Input: part model. Units: mm. Frame: model coordinates. Give positions to 0.01 mm unless a question says otherwise; leave off trailing zeros. Loops run counter-clockwise (first coordinate to the right, second up) from the corner with the lowest first, then second, coordinate; pieces in that order, holes last. Notation, with made-up numbers: (-28.5, 47.5) -> (-15.5, 47.5) arc R16 cw to (-15.5, 58.5) -> close; hole circle Ø10 at (59.5, -34.5). An arc over 180 degrees is marked (long way). Use CSV: the item, a comma, the result in double quotes.
```python
from build123d import *

# Parameters (mm, degrees)
F1_DEPTH = 18
F2_W     = 640.407225
F2_H     = 6
F3_DEPTH = 6


with BuildPart() as f1:
    # F0 (on Top) → F1 (new body)
    with BuildSketch(Plane.XY):
        Polygon((322.5, -311), (322.5, 311), (-322.5, 311), (-84.441184, -311), align=None)
    extrude(amount=F1_DEPTH)

    # F2 (on face) → F3 (cut)
    with BuildSketch(Plane.XY.offset(18)):
        with Locations((2.296388, 296)):
            Rectangle(F2_W, F2_H)
    extrude(amount=-F3_DEPTH, mode=Mode.SUBTRACT)


solid = f1.part
```
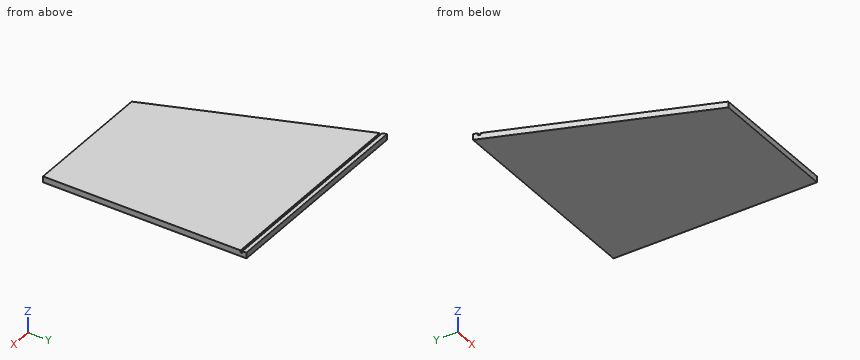
1) Section query A-A (x = -242). Return loops of the section in (y, z).
From the geometry:
outline,"(100.67, 0) -> (311, 0) -> (311, 18) -> (299, 18) -> (299, 12) -> (293, 12) -> (293, 18) -> (100.67, 18) -> close"
2) Section query C-C (y = -79). Return loops of the section in (x, z).
From the geometry:
outline,"(-173.23, 0) -> (322.5, 0) -> (322.5, 18) -> (-173.23, 18) -> close"
3) Section query B-B (z = 3). Return loops of the section in (x, y), then the cut area to 3 significant figures.
From the geometry:
outline,"(-322.5, 311) -> (-84.44, -311) -> (322.5, -311) -> (322.5, 311) -> close"
area,"327,000 mm^2"
4) Ray query, line 1 (Y direction, x = 89.5, z = 13); line 2 (X direction, y = 69, z = 9); line 3 (X direction, y = -11.5, z = 13.5). Return the intervals inside material, ascending.
From the geometry:
line 1,"y = -311 to 293, 299 to 311"
line 2,"x = -229.88 to 322.5"
line 3,"x = -199.07 to 322.5"
5) Contact query for a flat-ended pin moving along its axis: pin 1 (6 mm diameter, centred on y = 72.5, z = 3, fed in from -X). Output: stop coordinate, or through.
From the geometry:
pin 1,"stops at x = -232.37"
